Autodesk Fusion 360 part; units mm, degrees
sketch "Sketch1" plane through (0, 0, 0) normal (0, 0, 1) x (1, 0, 0)
  line L0 (-21, 11.5) -> (21, 11.5)
  line L1 (21, 11.5) -> (21, -11.5)
  line L2 (21, -11.5) -> (-21, -11.5)
  line L3 (-21, -11.5) -> (-21, 11.5)
  line L4 (-21, 11.5) -> (21, -11.5) construction
  line L5 (21, 11.5) -> (-21, -11.5) construction
  dimension "d1" = 42
  dimension "d2" = 23
extrude "Extrude1" add sketch "Sketch1" along normal blind 5
sketch "Sketch3" plane through (0, 0, 5) normal (0, 0, 1) x (-1, 0, 0)
  line L0 (21, 11.5) -> (-21, 11.5)
  line L1 (-21, 11.5) -> (-21, -11.5)
  line L2 (-21, -11.5) -> (21, -11.5)
  line L3 (21, -11.5) -> (21, 11.5)
  line L4 (-17.9148, 11.5098) -> (18.0852, 11.5098)
  line L5 (18.0852, 11.5098) -> (18.0852, 9.5098)
  line L6 (18.0852, 9.5098) -> (-17.9148, 9.5098)
  line L7 (-17.9148, 9.5098) -> (-17.9148, 11.5098)
  line L8 (-17.9148, 11.5098) -> (18.0852, 9.5098) construction
  line L9 (18.0852, 11.5098) -> (-17.9148, 9.5098) construction
  point P0 (0.0852, 10.5098)
  dimension "d44" = 36
  dimension "d45" = 2
extrude "Extrude3" add sketch "Sketch3" along normal blind 25 contours L0 L5 L6 L7 | L0 L4 L5 L7
sketch "Sketch4" plane through (0, 0, 30) normal (0, 0, 1) x (-1, 0, 0)
  line L0 (15, 10.5175) -> (-15, 10.5175)
  line L1 (-15, 10.5175) -> (-15, -13)
  line L2 (-15, -13) -> (15, -13)
  line L3 (15, -13) -> (15, 10.5175)
  line L4 (-17.9148, 9.5098) -> (18.0852, 9.5098)
  line L5 (18.0852, 9.5098) -> (18.0852, 11.5098)
  line L6 (18.0852, 11.5098) -> (-17.9148, 11.5098)
  line L7 (-17.9148, 11.5098) -> (-17.9148, 9.5098)
extrude "Extrude4" add sketch "Sketch4" along normal blind 2
ref_plane "WorkPlane1" through (21, 0, 5) normal (0.342, 0, 0.9397) x (0, 1, 0)
sketch "Sketch7" plane through (4.0635, 0, 11.1644) normal (0.342, 0, 0.9397) x (0, 1, 0)
  line L0 (-11.4455, -15.1007) -> (11.5394, -15.1007)
  line L1 (11.5394, -15.1007) -> (11.5394, -22.8179)
  line L2 (11.5394, -22.8179) -> (-11.4455, -22.8179)
  line L3 (-11.4455, -22.8179) -> (-11.4455, -15.1007)
extrude "Extrude7" add sketch "Sketch7" against normal blind 4.7
fillet "Fillet1" radius 3 2 edges at (24.7015, -11.4455, 1.1519) (24.7015, 11.5394, 1.1519)
fillet "Fillet2" radius 1 1 edges at (18.2536, 0.0469, 5.9996)
sketch "Sketch8" plane through (4.0635, 0, 11.1644) normal (0.342, 0, 0.9397) x (0, 1, 0)
  line L0 (11.5394, -16.1007) -> (-11.4455, -16.1007)
  line L1 (-8.4455, -22.8179) -> (8.5394, -22.8179)
  arc A0 (8.5394, -22.8179) -> (11.5394, -19.8179) centre (8.5394, -19.8179) ccw
  line L2 (11.5394, -19.8179) -> (11.5394, -16.1007)
  line L3 (-9, -17.0226) -> (9, -17.0226)
  line L4 (9, -17.0226) -> (9, -21.0226)
  line L5 (9, -21.0226) -> (-9, -21.0226)
  line L6 (-9, -21.0226) -> (-9, -17.0226)
  line L7 (-11.4455, -16.1007) -> (-11.4455, -18.0234)
  line L8 (-11.4455, -18.0234) -> (-11.4455, -19.8179)
  arc A1 (-11.4455, -19.8179) -> (-8.4455, -22.8179) centre (-8.4455, -19.8179) ccw
extrude "Extrude8" cut sketch "Sketch8" against normal blind 8 contours L3 L4 L5 L6
ref_plane "WorkPlane2" through (-21, 0, 5) normal (-0.342, 0, 0.9397) x (0, -1, 0)
sketch "Sketch9" plane through (4.0635, 0, 11.1644) normal (0.342, 0, 0.9397) x (0, 1, 0)
sketch "Sketch10" plane through (-4.0635, 0, 11.1644) normal (-0.342, 0, 0.9397) x (0, -1, 0)
  line L0 (11.4414, -15.0071) -> (-11.5436, -15.0071)
  line L1 (-11.5436, -15.0071) -> (-11.5436, -22.9991)
  line L2 (-11.5436, -22.9991) -> (11.4414, -22.9991)
  line L3 (11.4414, -22.9991) -> (11.4414, -15.0071)
  dimension "d29" = 22.985
  dimension "d30" = 7.992
extrude "Extrude9" add sketch "Sketch10" against normal blind 4.7
fillet "Fillet3" radius 3 2 edges at (-24.8718, -11.4414, 1.09) (-24.8718, 11.5436, 1.09)
sketch "Sketch11" plane through (4.0635, 0, 11.1644) normal (0.342, 0, 0.9397) x (0, 1, 0)
sketch "Sketch12" plane through (-4.0635, 0, 11.1644) normal (-0.342, 0, 0.9397) x (0, -1, 0)
  arc A0 (-11.5436, -19.9991) -> (-8.5436, -22.9991) centre (-8.5436, -19.9991) ccw
  line L0 (-8.5436, -22.9991) -> (8.4414, -22.9991)
  line L1 (11.4414, -19.9991) -> (11.4414, -18.0234)
  line L2 (11.4414, -15.0071) -> (-11.5436, -15.0071)
  line L3 (-11.5436, -15.0071) -> (-11.5436, -19.9991)
  line L4 (-9.1832, -17.1141) -> (8.8168, -17.1141)
  line L5 (8.8168, -17.1141) -> (8.8168, -21.1141)
  line L6 (8.8168, -21.1141) -> (-9.1832, -21.1141)
  line L7 (-9.1832, -21.1141) -> (-9.1832, -17.1141)
  arc A1 (8.4414, -22.9991) -> (11.4414, -19.9991) centre (8.4414, -19.9991) ccw
  line L8 (11.4414, -18.0234) -> (11.4414, -15.0071)
  dimension "d35" = 18
  dimension "d36" = 4
extrude "Extrude10" cut sketch "Sketch12" against normal blind 15 contours L4 L5 L6 L7
sketch "Sketch15" plane through (0, 13, 0) normal (0, 1, 0) x (-1, 0, 0)
  line L0 (-15, 30) -> (15, 30)
  line L1 (15, 30) -> (15, 32)
  line L2 (15, 32) -> (-15, 32)
  line L3 (-15, 32) -> (-15, 30)
  line L4 (-7, 32) -> (15, 32)
  line L5 (15, 32) -> (15, 23)
  line L6 (15, 23) -> (-7, 23)
  line L7 (-7, 23) -> (-7, 32)
extrude "Extrude12" add sketch "Sketch15" along normal blind 1 contours L0 L1 L2 L4 L5 L7 | L0 L5 L6 L7
fillet "Fillet4" radius 1 1 edges at (-18.1656, 0.0511, 6.0317)
ref_plane "WorkPlane3" through (0, -11.5, 0) normal (0, 1, 0) x (0, 0, 1)
sketch "Sketch18" plane through (0, -11.5, 0) normal (0, 1, 0) x (1, 0, 0)
  line L0 (-10, -32) -> (10, -32)
  line L1 (10, -32) -> (10, -37)
  line L2 (10, -37) -> (-10, -37)
  line L3 (-10, -37) -> (-10, -32)
extrude "Extrude13" add sketch "Sketch18" along normal blind 2
sketch "Sketch19" plane through (0, 0, 37) normal (0, 0, 1) x (-1, 0, 0)
  line L0 (10, 11.5) -> (-10, 11.5)
  line L1 (-10, 11.5) -> (-10, 9.5)
  line L2 (-10, 9.5) -> (10, 9.5)
  line L3 (10, 9.5) -> (10, 11.5)
  line L4 (10, 11.5) -> (-10, 11.5)
  line L5 (-10, 11.5) -> (-10, -9)
  line L6 (-10, -9) -> (10, -9)
  line L7 (10, -9) -> (10, 11.5)
extrude "Extrude14" add sketch "Sketch19" along normal blind 2
The listing builds one solid part. Answer for the finished solid, in the listing's coordinates (mm). A direction names the side the tool comes from. Give positions to 0.01 mm unless a question says otherwise; leave off trailing zeros. Write each loop counter-clockwise with the first axis right and the second up, starting at its lowest first coordinate (ties: lowest second). Pieces come first, ordered by that corner, then holes. Notation, with made-up numbers: (29, -15.75) -> (40, -15.75) arc R29 cw to (40, 6.25) -> close; hole circle Ø3 at (43, 41). An arc over 180 degrees is marked (long way). Write item = value, one per line. Start each with the question number.
1) Which of the six approach directions +Z, -Z, +X, -X, +Y, -Y give full straight-line access (tool end or side, diameter ignored) to faces 4 (the face through (23.026, 0.126, 1.797)), 5 (the face through (-15, 3, 31)), 6 (the face through (-22, -11.441, 3))?
2) Each of these flat-tipped pins is pushed along its axis until it touches: pin 1 (0.6 mm diameter, centred on x = -22, z = 3, fed in from -Y); pin 2 (6.5 mm diameter, centred on x = 18.5, z = 4, fed in from +Y); pin 3 (1.5 mm diameter, centred on x = -11.5, y = 0.5, fed in from +Z). Where does it stop, or does it pass through?
3) Straight lines are drawn through the part: line 1 along Z through (x, y) = (-4.5, -7.5); line 2 along Z through (x, y) = (-8.5, 9.75); line 3 along Y through (x, z) = (6.5, 28). For each, find the intervals that lie inside material, in ascending order.
4) Determine the mould class of faces 1 (the face through (-24.01, -10.59, 1.37)), 2 (the face through (-23.112, 0.057, 1.766)), 3 (the face through (0, 11.5, 2)) for opening direction Y: +Y half, -Y half, draft (parallel to the pull), parting line (faces both ways), or undercut.
5) The part is cut by section B-B, the plane y = 3. Determine the outline of the cut face in (x, z).
6) The part is cut by section A-A, the plane z = 28.5. Determine the outline of the cut face in (x, y).
7) The part is cut by section D-D, the plane z = 35.5. Determine the outline of the cut face in (x, y), and give its area (3 significant figures).
Solutions:
q1.face_4 = +Z
q1.face_5 = +Z, -X, +Y
q1.face_6 = +Z, -Z, -X, -Y
q2.pin_1 = -11.44
q2.pin_2 = 11.54
q2.pin_3 = 32
q3.line_1 = 0 to 5, 30 to 32, 37 to 39
q3.line_2 = 0 to 5, 30 to 32
q3.line_3 = -11.51 to -9.51, 13 to 14
q4.face_1 = -Y half
q4.face_2 = undercut
q4.face_3 = +Y half
q5.outline = (-25.68, 3.3) -> (-24.07, -1.12) -> (-22.3, -0.47) -> (-23.9, 3.94) -> close; (-20.15, 5.31) -> (-18.21, 0) -> (18.12, 0) -> (20.06, 5.34) -> (19.19, 5.66) arc R1 ccw to (17.91, 5.06) -> (17.89, 5) -> (-17.79, 5) -> (-17.82, 5.09) arc R1 ccw to (-19.11, 5.69) -> close; (-15, 30) -> (15, 30) -> (15, 32) -> (-15, 32) -> close; (-10, 37) -> (10, 37) -> (10, 39) -> (-10, 39) -> close; (22.21, -0.44) -> (23.9, -1.06) -> (25.51, 3.36) -> (23.82, 3.97) -> close
q6.outline = (-18.09, -11.51) -> (17.91, -11.51) -> (17.91, -9.51) -> (-18.09, -9.51) -> close; (-15, 13) -> (7, 13) -> (7, 14) -> (-15, 14) -> close
q7.outline = (-10, -11.5) -> (10, -11.5) -> (10, -9.5) -> (-10, -9.5) -> close
q7.area = 40.0 mm²
